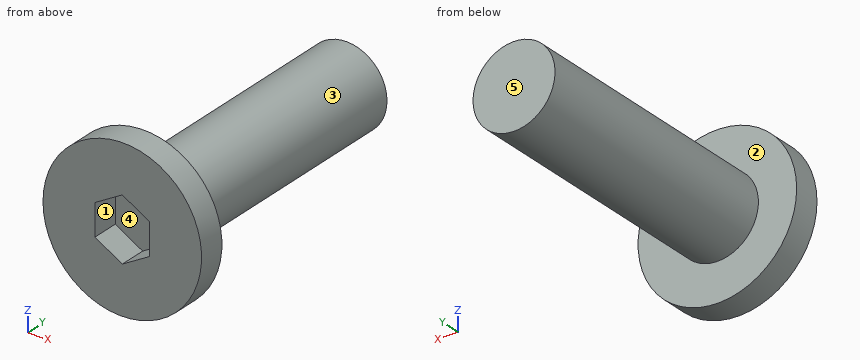
Autodesk Inventor part; units mm, degrees
ref_plane "YZ Plane" through (0, 0, 0) normal (1, 0, 0) x (0, 1, 0)
ref_plane "XZ Plane" through (0, 0, 0) normal (0, 1, 0) x (-1, 0, 0)
ref_plane "XY Plane" through (0, 0, 0) normal (0, 0, 1) x (1, 0, 0)
sketch "Sketch1" plane through (0, 0, 0) normal (0, 1, 0) x (-1, 0, 0)
  circle A0 centre (0, 0) radius 2.9
  dimension "d0" = 5.8
extrude "Extrusion1" add sketch "Sketch1" along normal blind 1
sketch "Sketch2" plane through (0, 1, 0) normal (0, 1, 0) x (1, 0, 0)
  circle A0 centre (0, 0) radius 1.5
  dimension "d3" = 3
extrude "Extrusion2" add sketch "Sketch2" along normal blind 10
sketch "Sketch3" plane through (0, 0, 0) normal (0, -1, 0) x (1, 0, 0)
  line L0 (0, -1.1547) -> (-1, -0.5774)
  line L1 (-1, -0.5774) -> (-1, 0.5774)
  line L2 (-1, 0.5774) -> (0, 1.1547)
  line L3 (0, 1.1547) -> (1, 0.5774)
  line L4 (1, 0.5774) -> (1, -0.5774)
  line L5 (1, -0.5774) -> (0, -1.1547)
  point P0 (0, 0)
  point P1 (0, 0)
  dimension "d6" = 2
extrude "Extrusion3" cut sketch "Sketch3" against normal blind 1
properties part number "m3_bolt_pan_8mm" material "Stainless Steel"
The model under review builds one solid part; all positions refer to its coordinate system, in mm. Face numbers are marked on the shaded views. A direction names the side the tool comes from. Coordinates: 2 decimals unless noted, no trailing zeros. Write each loop counter-clockwise with the first axis right and the second up, starting at its lowest first coordinate (ties: lowest second). Pieces come first, ordered by that corner, then holes. Notation, with made-up numbers: (35, -2) - (88, -2) arc R34 cw to (88, 35) - close; hole circle Ø3 at (73, 9). An arc over 180 degrees is marked (long way). Answer as a JSON object with one key per item and string values. Group by question number.
1. Add section A-A (z = 0). Give the boundary of the cut face in (x, y).
2. Add section C-C (y = 3.5). Give the boundary of the cut face in (x, z).
3. Add section D-D (x = -2.4). Give the boundary of the cut face in (y, z), plus the area to 3 significant figures.
4. Add section B-B (x = 0.4). Give the boundary of the cut face in (y, z), plus the area to 3 significant figures.
5. Clearance check with a flat-ended pin moving along its axis: pin 1 Ø1.5 at (x, y) = (-1.5, 5.5) entering from +Z. State where the tip first meets the part, or that it passes through.
6. To check wall thickness, follow probe 1 along Y at (x, z) = (-0.55, 0.1); probe 2 along Y at (x, z) = (-2.05, 1.3); probe 3 along X at (y, z) = (9.5, -1). State the ranges of each line that lie inside material, in increasing order.
7. Machinability: for the marked faces 4 and 5, which of the approach directions +Z, -Z, +X, -X, +Y, -Y give a long, thin tool a straight path to every point of the face, cutting with its end or side? Answer none if there is none.
8. Mouldability with a two-part tool opening along Z and no side actions: class the marked faces 1, 2 and 3 as pulls with the +Z half, pulls with the -Z half, needs draft (parallel to the pull), parting line crosses it, or undercut.
Findings:
{
 "1": {"outline": "(-2.9, 0) - (-1, 0) - (-1, 1) - (1, 1) - (1, 0) - (2.9, 0) - (2.9, 1) - (1.5, 1) - (1.5, 11) - (-1.5, 11) - (-1.5, 1) - (-2.9, 1) - close"},
 "2": {"outline": "circle Ø3 at (0, 0)"},
 "3": {"outline": "(0, -1.63) - (1, -1.63) - (1, 1.63) - (0, 1.63) - close", "area": "3.26 mm²"},
 "4": {"outline": "(0, -2.87) - (1, -2.87) - (1, -1.45) - (11, -1.45) - (11, 1.45) - (1, 1.45) - (1, 2.87) - (0, 2.87) - (0, 0.92) - (1, 0.92) - (1, -0.92) - (0, -0.92) - close", "area": "32.8 mm²"},
 "5": {"pin 1": "z = 1.3"},
 "6": {"probe 1": "1 to 11", "probe 2": "0 to 1", "probe 3": "-1.12 to 1.12"},
 "7": {"face 4": "-Y", "face 5": "+Z, -Z, +X, -X, +Y"},
 "8": {"face 1": "undercut", "face 2": "needs draft", "face 3": "parting line crosses it"}
}
